```python
from build123d import *

# Parameters (mm, degrees)
SKETCH1_W           = 9.525
SKETCH1_H           = 127
BOSS_EXTRUDE1_DEPTH = 24.13
SKETCH2_R           = 1.778
CUT_EXTRUDE1_DEPTH  = 10.525
SKETCH3_R           = 3.175
CUT_EXTRUDE2_DEPTH  = 38.1


with BuildPart() as part:
    # Sketch1 → Boss-Extrude1 (new body)
    with BuildSketch(Plane.XY):
        with Locations((4.7625, 63.5)):
            Rectangle(SKETCH1_W, SKETCH1_H)
    extrude(amount=BOSS_EXTRUDE1_DEPTH)

    # Sketch2 → Cut-Extrude1 (cut, through all)
    with BuildSketch(Plane.ZY):
        with Locations((5.9182, 101.6)):
            Circle(SKETCH2_R)
        with Locations((5.9182, 63.5)):
            Circle(SKETCH2_R)
        with Locations((5.9182, 25.4)):
            Circle(SKETCH2_R)
    extrude(amount=-CUT_EXTRUDE1_DEPTH, mode=Mode.SUBTRACT)

    # Sketch3 → Cut-Extrude2 (cut)
    with BuildSketch(Plane(origin=(9.525, 0, 0), x_dir=(0, 0, -1), z_dir=(1, 0, 0))):
        with Locations((-17.78, 63.5)):
            Circle(SKETCH3_R)
        with Locations((-17.78, 50.8)):
            Circle(SKETCH3_R)
    extrude(amount=-CUT_EXTRUDE2_DEPTH, mode=Mode.SUBTRACT)


solid = part.part
```
CAD build for the part. Positions are in the model's coordinates, mm. Round coordinates to 2 decimals unless told otherwise and drop trailing zeros. Order: outer loops, then holes, each group sorted by start corner. A loop starts at its lowest first (then second) coordinate and runs counter-clockwise, first axis right, second up.
Item 1: Saw through at B-B on z = 17.78. Write the cut outline in (x, y) (3 decimals), then the cut area to 3 significant figures.
Item 2: Saw through at C-C on x = 6.25. Write the cut outline in (y, z) (3 decimals).
Item 3: Mould opens along Z. For faces 1 (the face through (4.696, 100.023, 6.739)), 2 (the face through (5, 64, 24.13)), 3 (the face through (5, 127, 12)) say: pulls with the +Z half, pulls with the -Z half, needs draft (parallel to the pull), parting line crosses it, or undercut.
Item 4: Saw through at A-A on y = 63.5. Write the cut outline in (x, z) (3 decimals).
Item 5: Pin check, flat tip, straight feed: pin 1 (3 mm diameter, centred on y = 63.5, z = 5.92, fed in from -X). Stop position of the tip, or through.
Item 6: Probe line 1 along Y through (x, z) = (5.5, 18); line 2 along Y through (x, z) = (2, 20.5); line 3 along Z through (x, y) = (3.75, 101.6). List the from-to ranges inside material, lowest first.
Item 7: Saw through at D-D on y = 25.4. Write the cut outline in (x, z) (3 decimals), then the cut area to 3 significant figures.
Reported:
1. outline: (0, 0) - (9.525, 0) - (9.525, 47.625) - (0, 47.625) - close; (0, 53.975) - (9.525, 53.975) - (9.525, 60.325) - (0, 60.325) - close; (0, 66.675) - (9.525, 66.675) - (9.525, 127) - (0, 127) - close
1. area: 1,090 mm2
2. outline: (0, 0) - (127, 0) - (127, 24.13) - (0, 24.13) - close; hole circle Ø3.556 at (25.4, 5.918); hole circle Ø6.35 at (50.8, 17.78); hole circle Ø6.35 at (63.5, 17.78); hole circle Ø3.556 at (63.5, 5.918); hole circle Ø3.556 at (101.6, 5.918)
3. face 1: undercut
3. face 2: pulls with the +Z half
3. face 3: needs draft
4. outline: (0, 0) - (9.525, 0) - (9.525, 4.14) - (0, 4.14) - close; (0, 7.696) - (9.525, 7.696) - (9.525, 14.605) - (0, 14.605) - close; (0, 20.955) - (9.525, 20.955) - (9.525, 24.13) - (0, 24.13) - close
5. pin 1: passes through
6. line 1: y = 0 to 47.63, 53.97 to 60.33, 66.67 to 127
6. line 2: y = 0 to 49.16, 52.44 to 61.86, 65.14 to 127
6. line 3: z = 0 to 4.14, 7.7 to 24.13
7. outline: (0, 0) - (9.525, 0) - (9.525, 4.14) - (0, 4.14) - close; (0, 7.696) - (9.525, 7.696) - (9.525, 24.13) - (0, 24.13) - close
7. area: 196 mm2
